The model under review builds one solid part; all positions refer to its coordinate system, in mm. A direction names the side the tool comes from. Give positions to 0.01 mm unless a question says otherwise; leave off trailing zeros. Loops run counter-clockwise (first coordinate to the right, second up) from the corner with the lowest first, then second, coordinate; pieces in that order, holes last. Notation, with made-up numbers: M 78.25,44 L 132.25,44 A15 ccw 132.25,62 Z; hole C -17,-9.75 d6. An arc over 180 degrees is marked long. Write item = value, one per line. Start each with the question number.
1. Wall thickness on line 1 along X through (y, z) = (-5.25, 0); line 2 along Z through (x, y) = (0, -37); line 3 along Y through (x, z) = (8, 3.75): over which ranges is each line inside the solid? List them lowest first. Write a range as from..to.
2. We need section A-A on z = -9. Give the boundary of the cut face in (x, y).
3. For pin 1 (1.5 mm diameter, centred on y = -26, z = -1.5, fed in from +X); pin 2 (4 mm diameter, centred on x = 0, y = -5, fed in from -Z); pin 3 (6 mm diameter, centred on y = -25, z = 2, fed in from -X), all flat-tipped, find the tip position at first contact; note any pin that passes through.
4. We need section B-B on y = -36.5. Give the boundary of the cut face in (x, z).
5. We need section C-C on z = 5.75. Give the boundary of the cut face in (x, y).
6. Draft analysis for pull direction Z (two halves, no side actions). For faces 6 (the face through (0, -27.686, 0)), 7 (the face through (4.3, -14.24, 7.59)), 8 (the face through (-9, -0.711, 0)), 9 (the face through (0, -5, -8.496)), state which applies: pulls with the +Z half, pulls with the -Z half, needs draft (parallel to the pull), parting line crosses it, or undercut.
7. We need section D-D on x = 3.25. Give the boundary of the cut face in (y, z), then the cut area to 3 significant figures.
8. For faces 1 (the face through (-4.424, -14.24, 7.521)), 2 (the face through (-1.38, -34.69, 6.2)), 3 (the face through (-7.32, -4.73, -4.31)), 4 (the face through (-3, -15.85, -7)), 5 (the face through (-4.295, -25.226, -7.58)), list the 3-axis set-ups (+Z, -Z, +X, -X, +Y, -Y) from which the entire face can be reached by the end or side of a thin tool; tool diameter is ignored.
Autodesk Inventor part; units mm, degrees
ref_plane "YZ Plane" through (0, 0, 0) normal (1, 0, 0) x (0, 1, 0)
ref_plane "XZ Plane" through (0, 0, 0) normal (0, 1, 0) x (-1, 0, 0)
ref_plane "XY Plane" through (0, 0, 0) normal (0, 0, 1) x (1, 0, 0)
sketch "Sketch1" plane through (0, 0, 0) normal (0, 1, 0) x (-1, 0, 0)
  circle A0 centre (0, 0) radius 1.5875
  circle A1 centre (0, 0) radius 8.4963
  dimension "d0" = 3.175
  dimension "d1" = 16.9926
extrude "Extrusion1" add sketch "Sketch1" against normal blind 0.7112
sketch "Sketch2" plane through (0, -0.7112, 0) normal (0, -1, 0) x (1, 0, 0)
  circle A0 centre (0, 0) radius 8.4963 construction
  line L0 (4.9053, 8.4963) -> (9.8107, 0)
  line L1 (9.8107, 0) -> (4.9053, -8.4963)
  line L2 (4.9053, -8.4963) -> (-4.9053, -8.4963)
  line L3 (-4.9053, -8.4963) -> (-9.8107, 0)
  line L4 (-9.8107, 0) -> (-4.9053, 8.4963)
  line L5 (-4.9053, 8.4963) -> (4.9053, 8.4963)
  circle A1 centre (0, 0) radius 1.5875
  point P0 (0, 8.4963)
extrude "Extrusion2" add sketch "Sketch2" along normal blind 8.1534
sketch "Sketch3" plane through (0, -8.8646, 0) normal (0, -1, 0) x (1, 0, 0)
  circle A0 centre (0, 0) radius 8.2296
  dimension "d6" = 16.4592
extrude "Extrusion3" add sketch "Sketch3" along normal blind 3.81
sketch "Sketch4" plane through (0, -12.6746, 0) normal (0, -1, 0) x (1, 0, 0)
  circle A0 centre (0, 0) radius 8.7249 construction
  line L0 (8.7249, -5.0373) -> (0, -10.0746)
  line L1 (0, -10.0746) -> (-8.7249, -5.0373)
  line L2 (-8.7249, -5.0373) -> (-8.7249, 5.0373)
  line L3 (-8.7249, 5.0373) -> (0, 10.0746)
  line L4 (0, 10.0746) -> (8.7249, 5.0373)
  line L5 (8.7249, 5.0373) -> (8.7249, -5.0373)
  point P0 (8.7249, 0)
  dimension "d9" = 17.4498
extrude "Extrusion4" add sketch "Sketch4" along normal blind 3.175
sketch "Sketch5" plane through (0, -15.8496, 0) normal (0, -1, 0) x (1, 0, 0)
  circle A0 centre (0, 0) radius 7.112
  dimension "d12" = 14.224
extrude "Extrusion5" add sketch "Sketch5" along normal blind 6.985
sketch "Sketch6" plane through (0, -22.8346, 0) normal (0, -1, 0) x (1, 0, 0)
  circle A0 centre (0, 0) radius 8.7122 construction
  line L0 (8.7122, -5.03) -> (0, -10.06)
  line L1 (0, -10.06) -> (-8.7122, -5.03)
  line L2 (-8.7122, -5.03) -> (-8.7122, 5.03)
  line L3 (-8.7122, 5.03) -> (0, 10.06)
  line L4 (0, 10.06) -> (8.7122, 5.03)
  line L5 (8.7122, 5.03) -> (8.7122, -5.03)
  point P0 (8.7122, 0)
  dimension "d15" = 17.4244
extrude "Extrusion6" add sketch "Sketch6" along normal blind 4.8514
sketch "Sketch7" plane through (0, -27.686, 0) normal (0, -1, 0) x (1, 0, 0)
  circle A0 centre (0, 0) radius 2.4765
  circle A1 centre (0, 0) radius 6.35
  dimension "d18" = 4.953
  dimension "d19" = 12.7
extrude "Extrusion7" add sketch "Sketch7" along normal blind 14.1986
properties part number "am-2002" material "Brass"
Final values:
q1.line_1 = -9.81..-1.59, 1.59..9.81
q1.line_2 = -6.35..-2.48, 2.48..6.35
q1.line_3 = -27.69..-22.83, -15.85..-12.67
q2.outline = M -1.86,-15.85 L 1.86,-15.85 L 1.86,-12.67 L -1.86,-12.67 Z; M -1.84,-27.69 L 1.84,-27.69 L 1.84,-22.83 L -1.84,-22.83 Z
q3.pin_1 = 8.71
q3.pin_2 = -8.5
q3.pin_3 = -8.71
q4.outline = C 0,0 d12.7; hole C 0,0 d4.95
q5.outline = M -7.49,-15.85 L -4.19,-15.85 L -4.19,-22.83 L -7.47,-22.83 L -7.47,-27.69 L -2.69,-27.69 L -2.69,-41.88 L 2.69,-41.88 L 2.69,-27.69 L 7.47,-27.69 L 7.47,-22.83 L 4.19,-22.83 L 4.19,-15.85 L 7.49,-15.85 L 7.49,-12.67 L 5.89,-12.67 L 5.89,-8.86 L 6.49,-8.86 L 6.49,-0.71 L 6.25,-0.71 L 6.25,0 L -6.25,0 L -6.25,-0.71 L -6.49,-0.71 L -6.49,-8.86 L -5.89,-8.86 L -5.89,-12.67 L -7.49,-12.67 Z
q6.face_6 = undercut
q6.face_7 = pulls with the +Z half
q6.face_8 = needs draft
q6.face_9 = pulls with the -Z half
q7.outline = M -41.88,-5.46 L -27.69,-5.46 L -27.69,-8.18 L -22.83,-8.18 L -22.83,-6.33 L -15.85,-6.33 L -15.85,-8.2 L -12.67,-8.2 L -12.67,-7.56 L -8.86,-7.56 L -8.86,-8.5 L -0.71,-8.5 L -0.71,-7.85 L 0,-7.85 L 0,7.85 L -0.71,7.85 L -0.71,8.5 L -8.86,8.5 L -8.86,7.56 L -12.67,7.56 L -12.67,8.2 L -15.85,8.2 L -15.85,6.33 L -22.83,6.33 L -22.83,8.18 L -27.69,8.18 L -27.69,5.46 L -41.88,5.46 Z
q7.area = 582 mm²
q8.face_1 = +Z, -X, -Y
q8.face_2 = -Y
q8.face_3 = -Z, -X, +Y
q8.face_4 = none
q8.face_5 = -Z, -X, -Y
